Source: CAD feature listing. Evaluate the final solid. Frame: model axes, mm. Face numbers are marked on the shaded views. A direction names the side the tool comes from. Give positions to 0.01 mm unless a question says otherwise; leave off trailing zeros. Loops run counter-clockwise (first coordinate to the right, second up) from the corner with the lowest first, then second, coordinate; pieces in that order, holes last. Notation, with made-up numbers: M -33.5,-10 L 0.5,-10 A18 ccw 0.5,8 Z; hole C 11,41 d2. An arc over 180 degrees is marked long. Put each result on its own line as item: value. Start each with the question number.
```python
from build123d import *

# Parameters (mm, degrees)
F0_W     = 183.534793
F0_H     = 83.64898
F1_DEPTH = 15.056554
F2_R     = 5.08
F3_R     = 10.078833
F4_DEPTH = 140.712947


with BuildPart() as f1:
    # F0 (on Front) → F1 (new body)
    with BuildSketch(Plane.XZ):
        with Locations((0.603248, 41.82449)):
            Rectangle(F0_W, F0_H)
    extrude(amount=F1_DEPTH)

    # F2
    f2_edges = [f1.edges().sort_by_distance(p)[0] for p in [
        (0.603247, -15.056554, 83.64898),
        (-91.164149, -15.056554, 41.82449),
        (92.370644, -15.056554, 41.82449),
        (0.603247, -15.056554, 0),
    ]]
    fillet(f2_edges, radius=F2_R)

    # F3 (on face) → F4 (join)
    with BuildSketch(Plane.XZ.offset(15.056554)):
        with Locations((-49.689099, 46.704315)):
            Circle(F3_R)
    extrude(amount=F4_DEPTH)


solid = f1.part
```
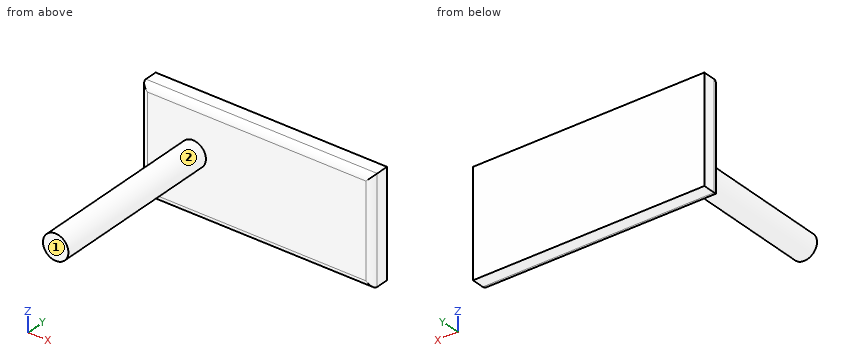
1. Section A-A, the plane z = 76. Output: boundary loops of the cut face in (x, y), plus the area to 3 significant figures.
2. Section D-D, the plane z = 50. Output: boundary loops of the cut face in (x, y).
3. Ray query, line 1 (Y direction, x = -5.5, z = 7.5); line 2 (X direction, y = -31, z = 47.5); line 3 (X direction, y = -45, z = 56). Return the intervals inside material, ascending.
4. Section B-B, the plane x = -63. Output: boundary loops of the cut face in (y, z).
5. Section C-C, the plane y = -106. Output: boundary loops of the cut face in (x, z).
6. Contact query for flat-ended pins moving along their axis: pin 1 (8 mm diameter, centred on y = -23.5, z = 35.5, fed in from +X); pin 2 (10 mm diameter, centred on x = -21, z = 75, fed in from -Y); pin 3 (4 mm diameter, centred on x = -55.5, y = -106, fed in from -Z). Output: stop coordinate, or through.
7. Set-up query: the marked faces 1 and 2. Return all of +Z, -Z, +X, -X, +Y, -Y with unobstructed straight access to the full face (end or side cutting, diameter ignored); none if empty.
Results found:
1. outline: M -91.16,-9.98 A5.08 ccw -86.08,-15.06 L 87.29,-15.06 A5.08 ccw 92.37,-9.98 L 92.37,0 L -91.16,0 Z
1. area: 2,750 mm²
2. outline: M -91.16,-9.98 A5.08 ccw -86.08,-15.06 L -59.21,-15.06 L -59.21,-155.77 L -40.16,-155.77 L -40.16,-15.06 L 87.29,-15.06 A5.08 ccw 92.37,-9.98 L 92.37,0 L -91.16,0 Z
3. line 1: -15.06 to 0
3. line 2: -59.74 to -39.64
3. line 3: -53.58 to -45.79
4. outline: M -15.06,5.08 A5.08 ccw -9.98,0 L 0,0 L 0,83.65 L -9.98,83.65 A5.08 ccw -15.06,78.57 Z
5. outline: C -49.69,46.7 d20.16
6. pin 1: x = -42.64
6. pin 2: y = -15.06
6. pin 3: z = 37.37
7. face 1: +Z, -Z, +X, -X, -Y
7. face 2: -Y
